```python
from build123d import *

# Parameters (mm, degrees)
CHAMFER1_SIZE      = 0.4
CUT_EXTRUDE1_DEPTH = 2


with BuildPart() as part:
    # Sketch1 → Revolve1 (revolve)
    with BuildSketch(Plane.XY):
        Polygon((-4, 0), (-4, 3.1), (-3.6, 3.5), (0, 3.5), (0, 2), (20, 2), (20, 0), align=None)
    revolve(axis=Axis((20, 0, 0), (-1, 0, 0)))

    # Chamfer1
    chamfer1_edges = [part.edges().sort_by_distance(p)[0] for p in [
        (20, -2, 0),
    ]]
    chamfer(chamfer1_edges, length=CHAMFER1_SIZE)

    # Sketch2 → Cut-Revolve1 (revolve, cut)
    with BuildSketch(Plane.XY):
        Polygon((-4, 0), (-4, 1.5), (-2, 1.5), (-1.598076211, 0), align=None)
    revolve(axis=Axis((-1.598076211, 0, 0), (-1, 0, 0)), mode=Mode.SUBTRACT)

    # Sketch3 → Cut-Extrude1 (cut)
    with BuildSketch(Plane(origin=(-4, 0, 0), x_dir=(0, 0, -1), z_dir=(1, 0, 0))):
        Polygon((-1.5, 0.866025404), (-1.5, -0.866025404), (0, -1.732050808), (1.5, -0.866025404), (1.5, 0.866025404), (0, 1.732050808), align=None)
    extrude(amount=CUT_EXTRUDE1_DEPTH, mode=Mode.SUBTRACT)


solid = part.part
```
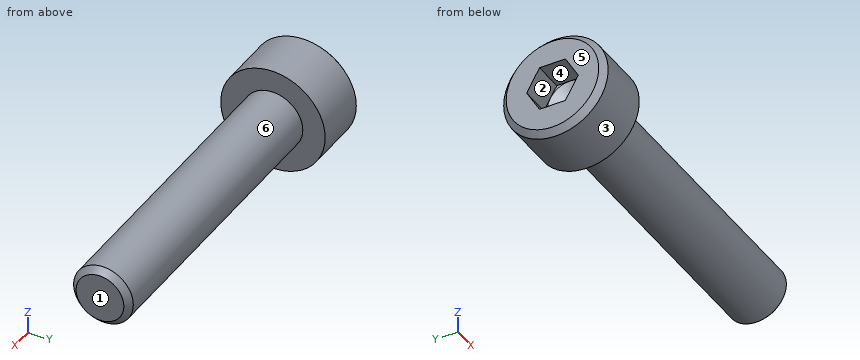
Check sheet for the modelled part. Datum: model origin and axes. Units: mm. Face numbers are marked on the shaded views. A direction names the side the tool comes from. Coordinates: 2 decimals unless noted, no trailing zeros. Order: outer loops, then holes, each group sorted by start corner. A loop starts at its lowest first (then second) coordinate and runs counter-clockwise, first axis right, second up. Notation, with made-up numbers: M 26.25,-10 L 44.25,-10 A19 cw 44.25,26 Z; hole C -4.5,46 d7. An arc over 180 degrees is marked long. Write each question's results on one line, items separated by ' | '. Start each with the question number.
1. Cross-section at A-A on x = 5. Record the cut outline in (y, z).
2. Go/stop test with flat-tipped pins: P1, Ø3, axis at x = 8, y = 1.5, coming from the -Z side; P2, Ø2, axis at x = 9, z = 2, coming from the -Y side; P3, Ø0.6, axis at y = 0.5, z = -1, coming from the -X side. Record where each tip stops, or that it passes through.
3. Access from +Z, -Z, +X, -X, +Y, -Y to the whole of each face (thin tool, end or side, straight path). Record for the marked faces 4, 5 and 6.
4. Mould release check, pull along Z, two halves, no side actions. Record for the marked faces 1, 2 and 3: +Z half, -Z half, draft (parallel to the pull), parting line (faces both ways), or undercut.
5. Material ranges on probe 1 along X at (y, z) = (1.5, 2.5); probe 2 along Y at (x, z) = (2, 1), recorded low to high.
Checks:
1) outline: C 0,0 d4
2) P1: stops at z = -2 | P2: stops at y = -1.73 | P3: stops at x = -1.98
3) face 4: -X | face 5: +Z, -Z, -X, +Y, -Y | face 6: +X
4) face 1: draft | face 2: undercut | face 3: parting line
5) probe 1: x = -4 to 0 | probe 2: y = -1.73 to 1.73
